Autodesk Inventor part; units mm, degrees
ref_plane "XZ Plane" through (0, 0, 0) normal (0, 1, 0) x (-1, 0, 0)
ref_plane "XY Plane" through (0, 0, 0) normal (0, 0, 1) x (1, 0, 0)
sketch "Sketch1" plane through (0, 0, 0) normal (0, 1, 0) x (-1, 0, 0)
  line L0 (76.2, 47.625) -> (-76.2, 47.625)
  line L1 (-76.2, 47.625) -> (-76.2, -47.625)
  line L2 (-76.2, -47.625) -> (76.2, -47.625)
  line L3 (76.2, -47.625) -> (76.2, 47.625)
  line L4 (76.2, 47.625) -> (-76.2, -47.625) construction
  line L5 (-76.2, 47.625) -> (76.2, -47.625) construction
  point P0 (0, 0)
  dimension "d0" = 152.4
  dimension "d1" = 95.25
extrude "Extrusion1" add sketch "Sketch1" against normal blind 6.35
sketch "Sketch4" plane through (0, 0, 0) normal (0, 1, 0) x (1, 0, 0)
  line L0 (-76.2, -19.05) -> (-57.15, -19.05)
  line L1 (-57.15, -19.05) -> (-57.15, 19.05)
  line L2 (-57.15, 19.05) -> (-76.2, 19.05)
  line L3 (-76.2, 19.05) -> (-76.2, -19.05)
  line L4 (-76.2, -19.05) -> (-57.15, 19.05) construction
  line L5 (-57.15, -19.05) -> (-76.2, 19.05) construction
  line L6 (-76.2, 47.625) -> (-76.2, -47.625)
  line L7 (-73.025, -15.875) -> (-60.325, -15.875)
  line L8 (-60.325, -15.875) -> (-60.325, 15.875)
  line L9 (-60.325, 15.875) -> (-73.025, 15.875)
  line L10 (-73.025, 15.875) -> (-73.025, -15.875)
  line L11 (-73.025, -15.875) -> (-60.325, 15.875) construction
  line L12 (-60.325, -15.875) -> (-73.025, 15.875) construction
  point P0 (0, 0)
  point P1 (-66.675, 0)
  dimension "d8" = 0
  dimension "d9" = 38.1
  dimension "d10" = 19.05
  dimension "d11" = 3.175
  dimension "d12" = 3.175
extrude "Extrusion2" add sketch "Sketch4" along normal blind 107.95
sketch "Sketch5" plane through (-76.2, -6.35, -47.625) normal (-1, 0, 0) x (0, 0, 1)
  circle A0 centre (47.625, 88.9) radius 4.7625
  line L0 (28.575, 114.3) -> (66.675, 114.3)
  line L1 (47.625, 6.35) -> (47.625, 114.3) construction
  dimension "d15" = 9.525
  dimension "d16" = 25.4
  dimension "d19" = 0
extrude "Extrusion3" cut sketch "Sketch5" against normal through all
mirror "Mirror1" about plane through (0, 0, 0) normal (1, 0, 0) of "Extrusion2", "Extrusion3"
equation "\"d0\" = baseWidth"
equation "\"d1\" = baseLength"
equation "\"d2\" = baseThickness"
equation "\"d9\" = postLength"
equation "\"d10\" = postWidth"
equation "\"d11\" = postWallThickness"
equation "\"d12\" = postWallThickness"
equation "\"d13\" = postHeight"
equation "\"d15\" = postAxelDiam"
equation "\"d16\" = heightFromTopToAxelCenter"
equation "\"d17\" = postHeight"
equation "\"baseWidth\" = 152.4"
equation "\"baseLength\" = 95.25"
equation "\"baseThickness\" = 6.35"
equation "\"postWidth\" = 19.05"
equation "\"postLength\" = 38.1"
equation "\"postWallThickness\" = 3.175"
equation "\"postAxelDiam\" = 9.525"
equation "\"heightFromTopToAxelCenter\" = 25.4"
equation "\"diamOfSproketPlusChain\" = 152.4"
equation "\"radiusOfSprocket\" = 0.5 * diamOfSproketPlusChain"
equation "\"heightOfAxelAboveBasePlate\" = radiusOfSprocket + gapBetweenChainAndBasePlate"
equation "\"gapBetweenChainAndBasePlate\" = 6.35"
equation "\"heightAboveRobotPlate\" = 50.8"
properties part number "MiddlePostsForTwoSprockets"
Design review of the part built by this model. Coordinates are the model's own, in mm. A direction names the side the tool comes from. Give positions to 0.01 mm unless a question says otherwise; leave off trailing zeros. Write each loop counter-clockwise with the first axis right and the second up, starting at its lowest first coordinate (ties: lowest second). Pieces come first, ordered by that corner, then holes. Notation, with made-up numbers: M 18.25,28.25 L 62.25,28.25 A24 ccw 62.25,64.25 Z; hole C 72,47 d3. An arc over 180 degrees is marked long. Answer as a JSON object with one key per item and string values. Group by question number.
1) Clearance check with flat-ended pins moving along their axes: pin 1 Ø14 at (x, y) = (64, 57) entering from +Z; pin 2 Ø10 at (x, y) = (65, 45) entering from -Z; pin 3 Ø10 at (x, z) = (-40, -18) entering from +Y; pin 4 Ø5.5 at (y, z) = (82.55, 0) entering from -X. State where each tip first meets the part, or that it passes through.
2) Tool access review of faces 5 (the face through (60.325, 53, 0)), 6 (the face through (74.63, 87.2, -1.03)), 7 (the face through (-67, 53, -19.05)), 8 (the face through (-57.15, 53, 0)), 9 (the face through (-67, 53, 19.05)): name each direction out of +Z, -Z, +X, -X, +Y, -Y from which nothing blocks a thin tool from reaching the whole face with its end or side.
3) We need section A-A (y = 101). Give the boundary of the cut face in (x, z) (3 decimals).
4) Mouldability with a two-part tool opening along Y and no side actions: class faces 1 (the face through (-73.2, 107.95, -0.3)), 2 (the face through (-58.76, 87.27, -0.62)), 3 (the face through (1, -6.35, 1)), 4 (the face through (-1, -3, 47.625)) as released by +Y, released by -Y, zero draft, split by the parting line, or undercut.
5) For line 1 along X through (y, z) = (40, 5) (3 decimals); line 2 along Y through (x, z) = (-75.4, 0); line 3 along X through (y, z) = (40, -17), list the stretches that pass through material, from the lowest coordinate up.
6) We need section B-B (z = 0). Count the separate pieces of the cut face and the enclosed holes in it, and give its area (3 significant figures).
7) We need section D-D (x = -35). Give the boundary of the cut face in (y, z) (3 decimals), and give its area (3 significant figures).
Answer key:
{
 "1": {"pin 1": "stops at z = 19.05", "pin 2": "stops at z = -19.05", "pin 3": "stops at y = 0", "pin 4": "passes through"},
 "2": {"face 5": "+Y", "face 6": "+X, -X", "face 7": "-Z, +X, -X, +Y", "face 8": "+Z, -Z, +Y", "face 9": "+Z, +X, -X, +Y"},
 "3": {"outline": "M -76.2,-19.05 L -57.15,-19.05 L -57.15,19.05 L -76.2,19.05 Z; M 57.15,-19.05 L 76.2,-19.05 L 76.2,19.05 L 57.15,19.05 Z; hole M -73.025,-15.875 L -60.325,-15.875 L -60.325,15.875 L -73.025,15.875 Z; hole M 60.325,-15.875 L 73.025,-15.875 L 73.025,15.875 L 60.325,15.875 Z"},
 "4": {"face 1": "released by +Y", "face 2": "undercut", "face 3": "released by -Y", "face 4": "zero draft"},
 "5": {"line 1": "x = -76.2 to -73.025, -60.325 to -57.15, 57.15 to 60.325, 73.025 to 76.2", "line 2": "y = -6.35 to 77.79, 87.31 to 107.95", "line 3": "x = -76.2 to -57.15, 57.15 to 76.2"},
 "6": {"separate pieces": "5", "enclosed holes": "0", "area": "2,220 mm²"},
 "7": {"outline": "M -6.35,-47.625 L 0,-47.625 L 0,47.625 L -6.35,47.625 Z", "area": "605 mm²"}
}
